```python
from build123d import *

# Parameters (mm, degrees)
BOSS_EXTRUDE1_DEPTH     = 5
CUT_EXTRUDE1_DEPTH      = 2
M2_5_CLEARANCE_HOLE1_D  = 2.9
RIB1_REACH              = 45.305
SKETCH5_WALL_W          = 114.10480654
SKETCH5_WALL_H          = 2
MIRROR2_COPY_1_REACH    = 45.305
MIRROR2_COPY_1_SKETCH_W = 114.10480654
MIRROR2_COPY_1_SKETCH_H = 2
CHAMFER1_SIZE           = 2
FILLET1_R               = 1


with BuildPart() as part:
    # Sketch1 → Boss-Extrude1 (new, symmetric)
    with BuildSketch(Plane(origin=(0, 0, 0), x_dir=(1, 0, 0), z_dir=(0, 1, 0))):
        Polygon((21.5, -19.5), (-21.5, -19.5), (-21.5, 19.5), (-34.5, 19.5), (-34.5, 14.5), (-26.5, 14.5), (-26.5, -24.188022284), (26.5, -24.188022284), (26.5, 14.5), (34.5, 14.5), (34.5, 19.5), (21.5, 19.5), align=None)
    extrude(amount=BOSS_EXTRUDE1_DEPTH, both=True)

    # Sketch2 → Cut-Extrude1 (cut)
    with BuildSketch(Plane.XY.offset(-14.5)):
        Polygon((-26.5, 1.5011107), (-29.1, 3.0022214), (-31.7, 1.5011107), (-31.7, -1.5011107), (-29.1, -3.0022214), (-26.5, -1.5011107), align=None)
    cut_extrude1 = extrude(amount=-CUT_EXTRUDE1_DEPTH, mode=Mode.SUBTRACT)

    # M2.5 Clearance Hole1 (through all)
    with Locations(Plane.XY.offset(-16.5)):
        with Locations((-29.1, 0)):
            m2_5_clearance_hole1 = Hole(M2_5_CLEARANCE_HOLE1_D / 2)

    # Sketch5 wall → Rib1 (add, up to next)
    with BuildSketch(Plane(origin=(-29, 5, -2), x_dir=(0.196116135138, 0, 0.980580675691), z_dir=(0.980580675691, 0, -0.196116135138)), mode=Mode.PRIVATE) as rib1_sk1:
        with Locations((0, 1)):
            Rectangle(SKETCH5_WALL_W, SKETCH5_WALL_H)
    rib1_tool1 = extrude(rib1_sk1.sketch, amount=RIB1_REACH, mode=Mode.PRIVATE) - part.part
    rib1 = rib1_tool1.solids().sort_by_distance((-29, 5, -2))[0]
    add(rib1)

    # Mirror1: Rib1 across plane
    add(rib1.mirror(Plane.ZX))

    # Mirror2: Cut-Extrude1, M2.5 Clearance Hole1, Rib1 across plane
    add(cut_extrude1.mirror(Plane(origin=(0, 0, 0), x_dir=(0, 0, 1), z_dir=(1, 0, 0))), mode=Mode.SUBTRACT)
    add(m2_5_clearance_hole1.mirror(Plane(origin=(0, 0, 0), x_dir=(0, 0, 1), z_dir=(1, 0, 0))), mode=Mode.SUBTRACT)
    add(rib1.mirror(Plane(origin=(0, 0, 0), x_dir=(0, 0, 1), z_dir=(1, 0, 0))))

    # Mirror2 copy 1 sketch → Mirror2 copy 1 (add, up to next)
    with BuildSketch(Plane(origin=(29, -5, -2), x_dir=(-0.196116135138, 0, 0.980580675691), z_dir=(-0.980580675691, 0, -0.196116135138)), mode=Mode.PRIVATE) as mirror2_copy_1_sk1:
        with Locations((0, 1)):
            Rectangle(MIRROR2_COPY_1_SKETCH_W, MIRROR2_COPY_1_SKETCH_H)
    mirror2_copy_1_tool1 = extrude(mirror2_copy_1_sk1.sketch, amount=MIRROR2_COPY_1_REACH, mode=Mode.PRIVATE) - part.part
    add(mirror2_copy_1_tool1.solids().sort_by_distance((29, -5, -2))[0])

    # Chamfer1
    chamfer1_edges = [part.edges().sort_by_distance(p)[0] for p in [
        (26.5, -2.25055535, -14.5),
        (26.5, 2.25055535, -14.5),
        (-26.5, -2.25055535, -14.5),
        (-26.5, 2.25055535, -14.5),
    ]]
    chamfer(chamfer1_edges, length=CHAMFER1_SIZE)

    # Fillet1
    fillet1_edges = [part.edges().sort_by_distance(p)[0] for p in [
        (-26.5, -5, 17.344011142),
        (-29, -5, -2),
        (-26.5, -3, -1),
        (-26.5, -4, 10.5),
        (0, -5, 24.188022284),
        (26.5, -1.5011107, -14.5),
        (26.5, 1.5011107, -14.5),
        (-34.5, -5, -17),
        (26.5, 0, -16.5),
        (34.5, 5, -17),
        (-21.5, -5, 0),
        (0, -5, 19.5),
        (21.5, -5, 0),
        (26.5, 5, 17.344011142),
        (34.5, -5, -17),
        (29, 5, -2),
        (26.5, 4, 10.5),
        (26.5, -5, 17.344011142),
        (26.5, -4, 10.5),
        (29, -5, -2),
        (26.5, 0, 24.188022284),
        (-26.5, 0, 24.188022284),
        (26.5, -3, -1),
        (-21.5, 0, -19.5),
        (-21.5, 0, 19.5),
        (21.5, 0, 19.5),
        (21.5, 0, -19.5),
        (21.5, 5, 0),
        (26.5, 3, -1),
        (26.5, 2.25055535, -12.5),
        (26.5, -2.25055535, -12.5),
        (-26.5, 3, -1),
        (-26.5, 2.25055535, -12.5),
        (-26.5, -2.25055535, -12.5),
        (0, 5, 19.5),
        (-21.5, 5, 0),
        (-26.5, 0, -16.5),
        (-26.5, 1.5011107, -14.5),
        (-26.5, -1.5011107, -14.5),
        (-34.5, 5, -17),
        (0, 5, 24.188022284),
        (-26.5, 5, 17.344011142),
        (-29, 5, -2),
        (-26.5, 4, 10.5),
    ]]
    fillet(fillet1_edges, radius=FILLET1_R)


solid = part.part
```
Model file for the job. Use its own axes, mm. A direction names the side the tool comes from. Round coordinates to 2 decimals unless told otherwise and drop trailing zeros. Loops run counter-clockwise (first coordinate to the right, second up) from the corner with the lowest first, then second, coordinate; pieces in that order, holes last. Notation, with made-up numbers: M 21,-14.5 L 46,-14.5 A37 ccw 46,23.5 Z; hole C 79.25,-23 d4. An arc over 180 degrees is marked long. Put each result on its own line as item: value. Start each with the question number.
Item 1: 3-axis set-ups, long thin cutter, end or side, ignore diameter. For faces 1 (the face through (-28.68, 4.715, -1.933)), 2 (the face through (-27, -2, -13)), 3 (the face through (27, -2, -13)), 4 (the face through (31, 0, -16.5)): which of +Z, -Z, +X, -X, +Y, -Y reach the whole face in a straight line?
Item 2: Drop flat-ended pins along their axis: P1, Ø1, axis at y = 0, z = 12, coming from the -X side; P2, Ø4.5, axis at x = -28.5, y = -1, coming from the +Z side; P3, Ø6, axis at y = 3, z = 9.5, coming from the +X side; P4, Ø1.7, axis at x = 29.1, y = 0, coming from the -Z side. Give the stop position or say it passes through.
Item 3: Drill centre lines: line 1 along X through (y, z) = (0.5, -8.5); line 2 along Y through (x, z) = (-29, -17); line 3 along X through (y, z) = (-1.5, -17). Where is each one in solid material? Low to high.
Item 4: Cut at A-A (y = 0). Give the number of separate pieces and of enclosed holes in the cut face, then the cut area to 3 significant figures.
Item 5: Cut at C-C (x = -7.5). List the corners of the cut face in (y, z).
Item 6: Mould opens along Y. For faces 5 (the face through (-31, 0, -16.5)), 6 (the face through (-27, 0, -19.5)), 7 (the face through (28.68, 4.715, -1.933)) say: released by +Y, released by -Y, zero draft, split by the parting line, or undercut.
Item 7: Cut at B-B (z = 13). List the corners of the cut face in (x, y).
Answer block:
1. face 1: +Z, -X, +Y
1. face 2: +Z, -X
1. face 3: +Z, +X
1. face 4: +Z
2. P1: x = -26.5
2. P2: z = 23.85
2. P3: x = 27.3
2. P4: through
3. line 1: -26.5 to -21.5, 21.5 to 26.5
3. line 2: -5 to -1.45, 1.45 to 5
3. line 3: -34.5 to -21.5, 21.5 to 34.5
4. separate pieces: 3
4. enclosed holes: 0
4. area: 680 mm2
5. outline: M -5,20.5 A1 ccw -4,19.5 L 4,19.5 A1 ccw 5,20.5 L 5,23.19 A1 ccw 4,24.19 L -4,24.19 A1 ccw -5,23.19 Z
6. face 5: undercut
6. face 6: zero draft
6. face 7: released by +Y
7. outline: M -26.5,-4 A1 ccw -25.5,-5 L -22.5,-5 A1 ccw -21.5,-4 L -21.5,4 A1 ccw -22.5,5 L -25.5,5 A1 ccw -26.5,4 Z; M 21.5,-4 A1 ccw 22.5,-5 L 25.5,-5 A1 ccw 26.5,-4 L 26.5,4 A1 ccw 25.5,5 L 22.5,5 A1 ccw 21.5,4 Z
